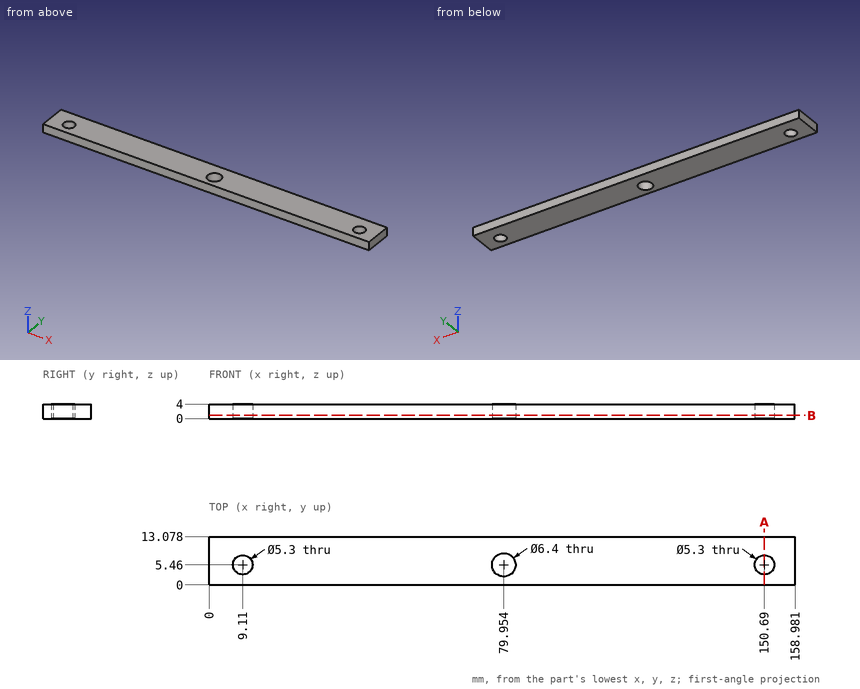
Drawing for the job (mm, zero at the part's lowest x, y, z). Give positions to 0.01 mm unless a question says otherwise; leave off trailing zeros. Loops run counter-clockwise (first coordinate to the right, second up) from the corner with the lowest first, then second, coordinate; pieces in that order, holes last.
Item 1: Drill centre lines: line 1 along Y through (x, z) = (9.5, 1.3); line 2 along X through (y, z) = (6.5, 2.5); line 3 along X through (y, z) = (4.25, 1.95) (1 decimal). Where is each one in solid material? Low to high.
Check values:
line 1: y = 0 to 2.84, 8.08 to 13.08
line 2: x = 0 to 6.67, 11.55 to 76.93, 82.98 to 148.25, 153.13 to 158.98
line 3: x = 0 to 6.8, 11.5 to 77, 82.9 to 148.3, 153 to 159
Item 2: Slice it at A-A (x = 150.69). Write the cut outline in (y, z), plus the area to 3 significant figures.
Check values:
outline: (0, 0) - (2.81, 0) - (2.81, 4) - (0, 4) - close; (8.11, 0) - (13.08, 0) - (13.08, 4) - (8.11, 4) - close
area: 31.1 mm2
Item 3: Slice it at B-B (z = 0.9). Write the cut outline in (x, y), plus the area to 3 significant figures.
Check values:
outline: (0, 0) - (158.98, 0) - (158.98, 13.08) - (0, 13.08) - close; hole circle Ø5.3 at (9.11, 5.46); hole circle Ø6.4 at (79.95, 5.46); hole circle Ø5.3 at (150.69, 5.46)
area: 2,000 mm2
